The model under review builds one solid part; all positions refer to its coordinate system, in mm. Face numbers are marked on the shaded views. A direction names the side the tool comes from. Give positions to 0.01 mm unless a question says otherwise; leave off trailing zeros. Order: outer loops, then holes, each group sorted by start corner. A loop starts at its lowest first (then second) coordinate and runs counter-clockwise, first axis right, second up. Notation, with made-up numbers: (40.5, 3) - (75.5, 3) arc R29 cw to (75.5, 32) - close; hole circle Ø9 at (-28, 34). An arc over 180 degrees is marked (long way). Use CSV: the item, a comma, the result in double quotes.
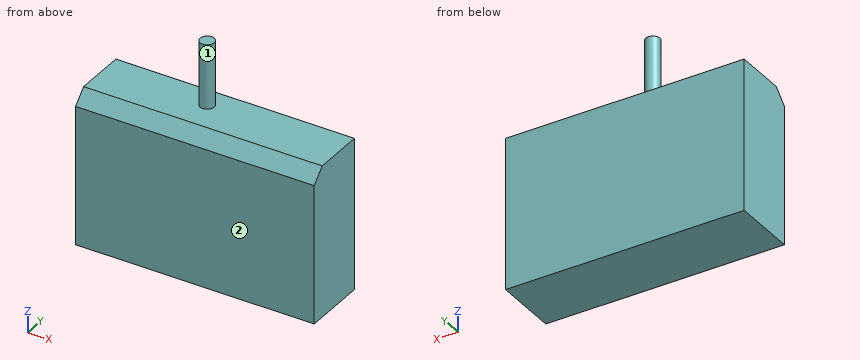
```python
from build123d import *

# Parameters (mm, degrees)
F0_W     = 93.8496552408
F0_H     = 59.6632584929
F1_DEPTH = 25.4
F2_SIZE  = 5.08
F3_R     = 2.779114803
F4_DEPTH = 25.4


with BuildPart() as f1:
    # F0 (on Front) → F1 (new body)
    with BuildSketch(Plane.XZ):
        with Locations((-7.3980521411, -0.1858584583)):
            Rectangle(F0_W, F0_H)
    extrude(amount=F1_DEPTH)

    # F2
    f2_edges = [f1.edges().sort_by_distance(p)[0] for p in [
        (-7.398052, -25.4, 29.645771),
    ]]
    chamfer(f2_edges, length=F2_SIZE)

    # F3 (on face) → F4 (join)
    with BuildSketch(Plane.XY.offset(29.6457707882)):
        with Locations((-13.2972076535, -8.1705600023)):
            Circle(F3_R)
    extrude(amount=F4_DEPTH)


solid = f1.part
```
Item 1: Take a section at D-D, the plane y = -21.5. Give the boundary of the cut face in (x, z), and give its area (3 significant figures).
Results list:
outline,"(-54.32, -30.02) - (39.53, -30.02) - (39.53, 28.47) - (-54.32, 28.47) - close"
area,"5,490 mm2"
Item 2: Clearance check with flat-ended pins moving along their axes: pin 1 (10 mm diameter, centred on x = -17, z = 29, fed in from -Y); pin 2 (12 mm diameter, centred on x = 22, y = -16, fed in from +Z). State where each tip first meets the part, or that it passes through.
Results list:
pin 1,"stops at y = -25.4"
pin 2,"stops at z = 29.65"
Item 3: Take a section at C-C, the plane z = 34. Give the boundary of the cut face in (x, y).
Results list:
outline,"circle Ø5.56 at (-13.3, -8.17)"
Item 4: Take a section at B-B, the plane y = -2.5. Give the boundary of the cut face in (x, z), and give its area (3 significant figures).
Results list:
outline,"(-54.32, -30.02) - (39.53, -30.02) - (39.53, 29.65) - (-54.32, 29.65) - close"
area,"5,600 mm2"
Item 5: Take a section at A-A, the plane x = 33. Give the boundary of the cut face in (y, z).
Results list:
outline,"(-25.4, -30.02) - (0, -30.02) - (0, 29.65) - (-20.32, 29.65) - (-25.4, 24.57) - close"
Item 6: Wall thickness on L1, parallel to Z at x = -25, y = -13.75; L2, parallel to X at y = -8.25, z = 43; L3, parallel to Z at x = -12, y = -21: over which ranges is each line inside the solid? List them lowest first.
Results list:
L1,"z = -30.02 to 29.65"
L2,"x = -16.08 to -10.52"
L3,"z = -30.02 to 28.97"
Item 7: Tool access review of the marked faces 1 and 2: name each direction out of +Z, -Z, +X, -X, +Y, -Y from which nothing blocks a thin tool from reaching the whole face with its end or side.
Results list:
face 1,"+Z"
face 2,"+Z, -Z, +X, -X, -Y"
